```python
from build123d import *

# Parameters (mm, degrees)
F1_DEPTH = 12.7
F2_T     = -2.54
F3_R     = 1.5875
F4_DEPTH = 10.16
F5_D     = 2.2606
F5_DEPTH = 10.161
F6_D     = 2.2606
F6_DEPTH = 10.161
F7_R     = 4.7625
F8_DEPTH = 25.4


with BuildPart() as f1:
    # F0 (on Top) → F1 (new body)
    with BuildSketch(Plane.XY):
        with BuildLine():
            ThreePointArc((-14.6767156663, 29.4530092287), (-12.0777332251, 26.6050755519), (-11.136649862, 22.8661187375))
            ThreePointArc((-11.136649862, 22.8661187375), (-14.7855906965, 16.2084748129), (-22.3607508211, 15.7025687681))
            ThreePointArc((-22.3607508211, 15.7025687681), (-18.0453134926, 8.9409904355), (-22.3607508211, 2.1794121029))
            ThreePointArc((-22.3607508211, 2.1794121029), (-14.7855906965, 1.673506058), (-11.136649862, -4.9841378665))
            ThreePointArc((-11.136649862, -4.9841378665), (-11.9647424889, -8.5047751532), (-14.2753729744, -11.287150229))
            ThreePointArc((-14.2753729744, -11.287150229), (-9.1296413708, -9.9591111779), (-4.06321014, -11.5633293799))
            ThreePointArc((-4.06321014, -11.5633293799), (-6.584769511, -1.1252359292), (3.6324394001, 2.1794121029))
            ThreePointArc((3.6324394001, 2.1794121029), (-0.6829979284, 8.9409904355), (3.6324394001, 15.7025687681))
            ThreePointArc((3.6324394001, 15.7025687681), (-6.588170937, 19.0132972903), (-4.0515957548, 29.4530092287))
            ThreePointArc((-4.0515957548, 29.4530092287), (-9.3641557105, 27.8546574286), (-14.6767156663, 29.4530092287))
        make_face()
        with BuildLine():
            ThreePointArc((-22.3607508211, 15.7025687681), (-14.7855906965, 16.2084748129), (-11.136649862, 22.8661187375))
            ThreePointArc((-11.136649862, 22.8661187375), (-12.0777332251, 26.6050755519), (-14.6767156663, 29.4530092287))
            ThreePointArc((-14.6767156663, 29.4530092287), (-25.9292475994, 26.7189401846), (-22.3607508211, 15.7025687681))
        make_face()
        with BuildLine():
            ThreePointArc((8.2044268003, 22.8661187375), (4.0453394351, 29.823079554), (-4.0515957548, 29.4530092287))
            ThreePointArc((-4.0515957548, 29.4530092287), (-6.588170937, 19.0132972903), (3.6324394001, 15.7025687681))
            ThreePointArc((3.6324394001, 15.7025687681), (6.9640265452, 18.6170153923), (8.2044268003, 22.8661187375))
        make_face()
        with BuildLine():
            ThreePointArc((-11.136649862, -4.9841378665), (-14.7855906965, 1.673506058), (-22.3607508211, 2.1794121029))
            ThreePointArc((-22.3607508211, 2.1794121029), (-25.8060038773, -9.0496593551), (-14.2753729744, -11.287150229))
            ThreePointArc((-14.2753729744, -11.287150229), (-11.9647424889, -8.5047751532), (-11.136649862, -4.9841378665))
        make_face()
        with BuildLine():
            ThreePointArc((8.2044268003, -4.9841378665), (6.9640265452, -0.7350345214), (3.6324394001, 2.1794121029))
            ThreePointArc((3.6324394001, 2.1794121029), (-6.584769511, -1.1252359292), (-4.06321014, -11.5633293799))
            ThreePointArc((-4.06321014, -11.5633293799), (4.0392009389, -11.9443942747), (8.2044268003, -4.9841378665))
        make_face()
    extrude(amount=F1_DEPTH)

    # F2
    f2_openings = [f1.faces().sort_by_distance(p)[0] for p in [
        (-9.363943, 8.943821, 12.7),
    ]]
    offset(amount=F2_T, openings=f2_openings, kind=Kind.INTERSECTION)

    # F3 (on face) → F4 (join, through all)
    with BuildSketch(Plane.XY.offset(2.54)):
        with Locations((-19.0346940417, 22.8661187375)):
            Circle(F3_R)
        with Locations((0.3063826207, 22.8661187375)):
            Circle(F3_R)
        with Locations((-19.0346940417, -4.9841378665)):
            Circle(F3_R)
        with Locations((0.3063826207, -4.9841378665)):
            Circle(F3_R)
    extrude(amount=F4_DEPTH)

    # F5 (through all, one way)
    with BuildSketch(Plane(origin=(0, 0, 2.54), x_dir=(1, 0, 0), z_dir=(0, 0, -1))):
        with Locations((-19.0346940417, -22.8661187375)):
            Circle(F5_D / 2)
    extrude(amount=-F5_DEPTH, mode=Mode.SUBTRACT)

    # F6 (through all, one way)
    with BuildSketch(Plane(origin=(0, 0, 2.54), x_dir=(1, 0, 0), z_dir=(0, 0, -1))):
        with Locations((0.3063826207, -22.8661187375), (0.3063826207, 4.9841378665), (-19.0346940417, 4.9841378665)):
            Circle(F6_D / 2)
    extrude(amount=-F6_DEPTH, mode=Mode.SUBTRACT)

    # F7 (on Front) → F8 (cut)
    with BuildSketch(Plane.XZ):
        with Locations((-9.3144346029, 12.7)):
            Circle(F7_R)
    extrude(amount=F8_DEPTH, mode=Mode.SUBTRACT)


solid = f1.part
```
Check sheet for the modelled part. Datum: model origin and axes. Units: mm. A direction names the side the tool comes from. Round coordinates to 2 decimals unless told otherwise and drop trailing zeros. Loops run counter-clockwise (first coordinate to the right, second up) from the corner with the lowest first, then second, coordinate; pieces in that order, holes last. Notation, with made-up numbers: (62.25, 87) - (120.25, 87) arc R14 ccw to (120.25, 101) - close; hole circle Ø2 at (40.5, 64.25). An arc over 180 degrees is marked (long way). Write item = value, one per line. Start each with the question number.
Q1. Section check C-C (x = -6). Record the boundary of the cut face in (y, z).
Q2. Section check B-B (y = 19). Record the boundary of the cut face in (x, z).
Q3. Thickness scan on L1, parallel to Y at x = 3, z = 11.25; L2, parallel to Y at x = -1.5, z = 11; L3, parallel to Y at x = 2, z = 4.5. Record the ranges inside material, lowest first.
Q4. Release check for a two-part mould opening along Y. For faces 4 (the face through (-20, -6, 12.7)), 5 (the face through (-9.285, 27.855, 6.261)), 6 (the face through (0.159, -6.105, 7.549)) record: pulls with the +Y half, pulls with the -Y half, needs draft (parallel to the pull), parting line crosses it, or undercut.
Q5. Access from +Z, -Z, +X, -X, +Y, -Y to the whole of each face (thin tool, end or side, straight path). Record for faces 1 (the face through (-9.42, -9.31, 7.94)), 2 (the face through (-23.65, 25.59, 7.55)), 3 (the face through (-18.046, 9.06, 6.261)).
Q6. Section check A-A (z = 6.5). Count the separate pieces of the cut face and the enclosed holes in it, plus the area to 3 significant figures.
Q7. Depth check by flat-ended pin: P1, Ø2, axis at y = 0, z = 5.5, coming from the -X side; P2, Ø1.1, axis at x = 0, y = 22.5, coming from the +Z side; P3, Ø5, axis at y = 18.5, z = 5, coming from the +X side. Enter the tip coordinate at first touch or a pass-through.
Derived:
q1.outline = (-10.57, 0) - (28.46, 0) - (28.46, 12.7) - (25.79, 12.7) - (25.79, 2.54) - (-7.9, 2.54) - (-7.9, 9.28) - (-10.57, 9.28) - close
q2.outline = (-25.92, 0) - (7.19, 0) - (7.19, 12.7) - (4.02, 12.7) - (4.02, 2.54) - (-22.74, 2.54) - (-22.74, 12.7) - (-25.92, 12.7) - close
q3.L1 = -12.41 to -9.62, -0.35 to 2.51, 15.37 to 18.23, 27.5 to 30.29
q3.L2 = -12.67 to -10.03, 3.33 to 14.55, 27.91 to 30.55
q3.L3 = -12.7 to -10.07, 0.16 to 3.21, 14.67 to 17.72, 27.95 to 30.58
q4.face_4 = needs draft
q4.face_5 = pulls with the +Y half
q4.face_6 = undercut
q5.face_1 = +Z, -Y
q5.face_2 = +Z
q5.face_3 = +Z, -Z, -X
q6.separate_pieces = 5
q6.enclosed_holes = 5
q6.area = 403 mm^2
q7.P1 = -25.85
q7.P2 = 2.54
q7.P3 = 7.98
